Model file for the job. Use its own axes, mm. A direction names the side the tool comes from. Give positions to 0.01 mm unless a question says otherwise; leave off trailing zeros. Order: outer loops, then holes, each group sorted by start corner. A loop starts at its lowest first (then second) coordinate and runs counter-clockwise, first axis right, second up. Notation, with made-up numbers: M -19.75,-1 L 2.25,-1 A8 ccw 2.25,10 Z; hole C 5.5,68 d6. An arc over 180 degrees is marked long. Return JSON: item names as keys, results as strings. Group by question number.
1. Slice it at A-A on y = -8. List the corners of the cut face in (x, z), then the cut area to 3 significant figures.
2. 3-axis set-ups, long thin cutter, end or side, ignore diameter. For faces 4 (the face through (0.33, 0.227, 7.493)), 5 (the face through (-3.955, -22.007, 5.158)), 6 (the face through (-3.955, 21.993, 5.158)), 7 (the face through (7.09, 16.88, 0.93)): which of +Z, -Z, +X, -X, +Y, -Y reach the whole face in a straight line?
3. Wall check: probe 1 along Y at (x, z) = (5.75, -3.75); probe 2 along Y at (x, z) = (6.75, 2.5); probe 3 along X at (y, z) = (-22.05, 0). Give the ranges that are in metal, low to high. Write a range as [from, to].
4. Two-plate mould, pull along Z, no slides. Class faces 1 (the face through (-6, -22.5, 3)), 2 (the face through (0.33, 19.858, 7.493)), 3 (the face through (7.04, -21.01, 0.92)): released by +Z, released by -Z, zero draft, split by the parting line, or undercut.
5. Pin check, flat tips, straight feed: pin 1 (4.5 mm diameter, centred on x = 2, z = -2.5, fed in from +Y); pin 2 (7 mm diameter, centred on x = 3, z = -1.5, fed in from -Y); pin 3 (3 mm diameter, centred on x = -3.5, z = 3.5, fed in from -Y); pin 4 (3 mm diameter, centred on x = 3.5, y = 12, fed in from -Z). Stop position of each tip, or through.
6. Slice it at B-B on y = -17. List the corners of the cut face in (x, z), then the cut area to 3 significant figures.
from build123d import *


with BuildPart() as part:
    # Sketch1 → Revolve1 (revolve)
    with BuildSketch(Plane(origin=(0, 0, 0), x_dir=(0, -1, 0), z_dir=(1, 0, 0))):
        with BuildLine():
            Line((-17.5, 7.5), (-22.15, 7.5))
            ThreePointArc((-22.15, 7.5), (-22.397487373, 7.397487373), (-22.5, 7.15))
            Line((-22.5, 7.15), (-22.5, 6.5))
            Line((-22.5, 6.5), (-21.5, 6.5))
            Line((-21.5, 6.5), (-21.5, 7.1))
            Line((-21.5, 7.1), (-20.5, 7.1))
            Line((-20.5, 7.1), (-20.5, 5.5))
            Line((-20.5, 5.5), (20.5, 5.5))
            Line((20.5, 5.5), (20.5, 7.1))
            Line((20.5, 7.1), (21.5, 7.1))
            Line((21.5, 7.1), (21.5, 6.5))
            Line((21.5, 6.5), (22.5, 6.5))
            Line((22.5, 6.5), (22.5, 7.15))
            ThreePointArc((22.5, 7.15), (22.397487373, 7.397487373), (22.15, 7.5))
            Line((22.15, 7.5), (17.5, 7.5))
            Line((17.5, 7.5), (17.5, 7.15))
            Line((17.5, 7.15), (16.25, 7.15))
            Line((16.25, 7.15), (16.25, 7.5))
            Line((16.25, 7.5), (-16.25, 7.5))
            Line((-16.25, 7.5), (-16.25, 7.15))
            Line((-16.25, 7.15), (-17.5, 7.15))
            Line((-17.5, 7.15), (-17.5, 7.5))
        make_face()
    revolve(axis=Axis((0, 12, 0), (0, -1, 0)))


solid = part.part
Result:
{
 "1": {"outline": "C 0,0 d15; hole C 0,0 d11", "area": "81.7 mm2"},
 "2": {"face 4": "+Y, -Y", "face 5": "-Y", "face 6": "+Y", "face 7": "none"},
 "3": {"probe 1": "y = [-22.5, -21.5], [-20.5, 20.5], [21.5, 22.5]", "probe 2": "y = [-22.5, -17.5], [-16.25, 16.25], [17.5, 22.5]", "probe 3": "x = [-7.5, -6.5], [6.5, 7.5]"},
 "4": {"face 1": "zero draft", "face 2": "split by the parting line", "face 3": "undercut"},
 "5": {"pin 1": "passes through", "pin 2": "stops at y = -22.5", "pin 3": "stops at y = -20.5", "pin 4": "stops at z = -7.23"},
 "6": {"outline": "C 0,0 d14.3; hole C 0,0 d11", "area": "65.6 mm2"}
}
